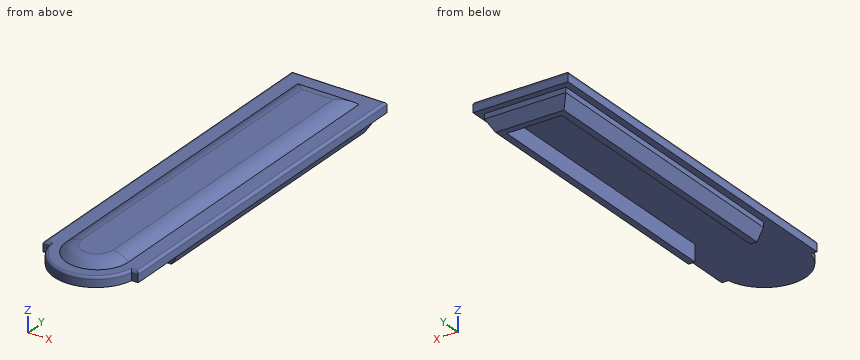
from build123d import *

# Parameters (mm, degrees)
F1_DEPTH    = 3
F3_DEPTH    = 5
F4_SIZE2    = 3.4641016151
F4_SIZE     = 2
F6_DEPTH    = 2
F6_TAPER    = 25
F7_T1_DEPTH = 109.1731798991
F7_T3_DEPTH = 35.3291597983
F7_T6_ANGLE = 180
F8_R        = 0.762


# Not quite as in the source:
# - a fillet or chamfer that OpenCascade refuses, or shapes differently, is made with other operations: its cross-section is extruded or revolved along the edge and cut away or added


with BuildPart() as f1:
    # F0 (on Top) → F1 (new body)
    with BuildSketch(Plane.XY):
        with BuildLine():
            Line((28.7274, 108.839), (0, 108.839))
            Line((0, 108.839), (0, 0))
            Line((0, 0), (1.9812, 0))
            ThreePointArc((1.9812, 0), (14.3637, -10.287), (26.7462, 0))
            Line((26.7462, 0), (28.7274, 0))
            Line((28.7274, 0), (28.7274, 108.839))
        make_face()
    extrude(amount=F1_DEPTH)

    # F2 (on face) → F3 (join)
    with BuildSketch(Plane(origin=(0, 0, 0), x_dir=(1, 0, 0), z_dir=(0, 0, -1))):
        Polygon((6.032, -20.447), (2.032, -20.447), (2.032, -106.807), (26.6954, -106.807), (26.6954, -20.447), (22.6954, -20.447), (22.6954, -102.807), (6.032, -102.807), align=None)
    extrude(amount=F3_DEPTH)

    # F4
    f4_edges = [f1.edges().sort_by_distance(p)[0] for p in [
        (2.032, 63.627, -5),
        (14.3637, 106.807, -5),
        (26.6954, 63.627, -5),
    ]]
    f4_side = f1.faces().sort_by_distance((4.032, 21.345128, -5))[0]
    chamfer(f4_edges, length=F4_SIZE, length2=F4_SIZE2, reference=f4_side)

    # F5 (on face) → F6 (join)
    with BuildSketch(Plane.XY.offset(3)):
        with BuildLine():
            Line((23.7274, 103.839), (5, 103.839))
            Line((5, 103.839), (5, 2.9667))
            ThreePointArc((5, 2.9667), (14.3637, -6.397), (23.7274, 2.9667))
            Line((23.7274, 2.9667), (23.7274, 103.839))
        make_face()
    extrude(amount=F6_DEPTH, taper=F6_TAPER)

    # F7: fillet of radius 6.35 on 4 edges, made by hand

    # F7_s2 → F7_t1 (cut)
    with BuildSketch(Plane.XZ.offset(-112.1398798991)):
        with BuildLine():
            ThreePointArc((23.7274, 3), (21.6213072312, 4.4785933123), (19.1013865975, 5))
            Line((19.1013865975, 5), (22.7947846837, 5))
            Line((22.7947846837, 5), (23.7274, 3))
        make_face()
        with BuildLine():
            ThreePointArc((5, 3), (7.1060927688, 4.4785933123), (9.6260134025, 5))
            Line((9.6260134025, 5), (5.9326153163, 5))
            Line((5.9326153163, 5), (5, 3))
        make_face()
    extrude(amount=F7_T1_DEPTH, mode=Mode.SUBTRACT)

    # F7_s4 → F7_t3 (cut)
    with BuildSketch(Plane.YZ.offset(-3.3008798991)):
        with BuildLine():
            ThreePointArc((103.839, 3), (101.7329072312, 4.4785933123), (99.2129865975, 5))
            Line((99.2129865975, 5), (102.9063846837, 5))
            Line((102.9063846837, 5), (103.839, 3))
        make_face()
    extrude(amount=F7_T3_DEPTH, mode=Mode.SUBTRACT)

    # F7_s5 → F7_t6 (revolve, cut)
    with BuildSketch(Plane.XZ.offset(-2.9667)):
        with BuildLine():
            ThreePointArc((5, 3), (7.1060927688, 4.4785933123), (9.6260134025, 5))
            Line((9.6260134025, 5), (5.9326153163, 5))
            Line((5.9326153163, 5), (5, 3))
        make_face()
    revolve(axis=Axis((14.3637, 2.9667, 5), (0, 0, 1)), revolution_arc=F7_T6_ANGLE, mode=Mode.SUBTRACT)

    # F8
    f8_edges = [f1.edges().sort_by_distance(p)[0] for p in [
        (0, 54.4195, 3),
        (0.9906, 0, 3),
        (14.3637, -10.287, 3),
        (27.7368, 0, 3),
        (28.7274, 54.4195, 3),
        (14.3637, 108.839, 3),
    ]]
    fillet(f8_edges, radius=F8_R)


solid = f1.part
Geometry check sheet. Reference: the model listing, model coordinates, mm. Round coordinates to 2 decimals unless told otherwise and drop trailing zeros. Loops run counter-clockwise (first coordinate to the right, second up) from the corner with the lowest first, then second, coordinate; pieces in that order, holes last.
Item 1: Cross-section at A-A on y = 85. Record the boundary of the cut face in (x, z), then the cut area to 3 significant figures.
Item 2: Thickness scan on line 1 (X direction, y = 37, z = -1.5); line 2 (Z direction, x = 12.5, y = 71); line 3 (Y direction, x = 25, z = -0.25). Record the ranges inside material, lowest first.
Item 3: Gauge pin test, flat ends, axial feed: pin 1 (1 mm diameter, centred on x = 5, z = 0, fed in from -Y); pin 2 (6 mm diameter, centred on x = 7, z = -2, fed in from -Y); pin 3 (1 mm diameter, centred on x = 13.5, y = 84.5, fed in from -Z). Record the tip position at first contact, or that the pin passes through.
Item 4: Cross-section at D-D on z = -3.25. Record the boundary of the cut face in (x, y).
Item 5: Cross-section at B-B on z = 1.25. Record the boundary of the cut face in (x, y), then the cut area to 3 significant figures.
Item 6: Cross-section at C-C on y = 5.5. Record the boundary of the cut face in (x, z), then the cut area to 3 significant figures.
Answer sheet:
1. outline: (0, 0) - (2.03, 0) - (2.03, -1.54) - (4.03, -5) - (6.03, -5) - (6.03, 0) - (22.7, 0) - (22.7, -5) - (24.7, -5) - (26.7, -1.54) - (26.7, 0) - (28.73, 0) - (28.73, 2.24) arc R0.76 ccw to (27.97, 3) - (23.73, 3) arc R6.35 ccw to (19.1, 5) - (9.63, 5) arc R6.35 ccw to (5, 3) - (0.76, 3) arc R0.76 ccw to (0, 2.24) - close
1. area: 151 mm2
2. line 1: x = 2.03 to 6.03, 22.7 to 26.7
2. line 2: z = 0 to 5
2. line 3: y = 20.45 to 106.81
3. pin 1: stops at y = -6.64
3. pin 2: stops at y = -9.2
3. pin 3: stops at z = 0
4. outline: (3.02, 20.45) - (6.03, 20.45) - (6.03, 102.81) - (22.7, 102.81) - (22.7, 20.45) - (25.71, 20.45) - (25.71, 105.82) - (3.02, 105.82) - close
5. outline: (0, 0) - (1.98, 0) arc R12.6 ccw to (26.75, 0) - (28.73, 0) - (28.73, 108.84) - (0, 108.84) - close
5. area: 3,320 mm2
6. outline: (0, 0) - (28.73, 0) - (28.73, 2.24) arc R0.76 ccw to (27.97, 3) - (23.73, 3) arc R6.35 ccw to (19.1, 5) - (9.63, 5) arc R6.35 ccw to (5, 3) - (0.76, 3) arc R0.76 ccw to (0, 2.24) - close
6. area: 118 mm2
